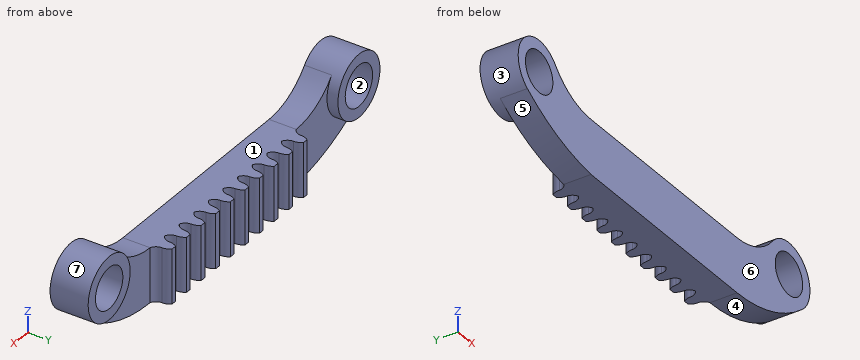
from build123d import *

# Parameters (mm, degrees)
SKETCH1_R                       = 3.75
BOSS_EXTRUDE1_DEPTH             = 5
BOSS_EXTRUDE2_REACH             = 43.932
SKETCH2_W                       = 1
SKETCH2_H                       = 1.5
BOSS_EXTRUDE2_DIRECTION_2_REACH = 43.932
LPATTERN1_COUNT                 = 10
LPATTERN1_PITCH                 = 4
SKETCH1_3_R                     = 5.75
SKETCH1_3_R_2                   = 3.75
BOSS_EXTRUDE3_DEPTH             = 7


with BuildPart() as part:
    # Sketch1 → Boss-Extrude1 (new body)
    with BuildSketch(Plane(origin=(0, 0, 0), x_dir=(1, 0, 0), z_dir=(0, 1, 0))):
        with BuildLine():
            ThreePointArc((-37.419913953, -1.242883661), (-38.427487159, -9.886669857), (-29.729020754, -9.627969703))
            ThreePointArc((-29.729020754, -9.627969703), (-25.386834609, -6.215943245), (-20, -5))
            Line((-20, -5), (20, -5))
            ThreePointArc((20, -5), (25.386834609, -6.215943245), (29.729020754, -9.627969703))
            ThreePointArc((29.729020754, -9.627969703), (38.202781159, -10.118262664), (37.932471123, -1.634635193))
            ThreePointArc((37.932471123, -1.634635193), (29.560228877, 3.288161479), (20, 5))
            Line((20, 5), (-20, 5))
            ThreePointArc((-20, 5), (-29.105909857, 2.983410588), (-37.419913953, -1.242883661))
        make_face()
        with Locations(Location((-34.19, -6, 0), (0, 0, 270))):
            Circle(SKETCH1_R, mode=Mode.SUBTRACT)
        with Locations(Location((34.19, -6, 0), (0, 0, 270))):
            Circle(SKETCH1_R, mode=Mode.SUBTRACT)
    extrude(amount=BOSS_EXTRUDE1_DEPTH)

    # Boss-Extrude2: up to this face of the body (flat: up to its plane)
    boss_extrude2_end = Plane(part.part.faces().sort_by_distance((0, 2.5, 5))[0])
    # Sketch2 → Boss-Extrude2 (add, up to the picked face)
    with BuildSketch(Plane.XY, mode=Mode.PRIVATE) as boss_extrude2_sk1:
        with BuildLine():
            ThreePointArc((-19, 6.5), (-19.272918272, 5.598612181), (-20, 5))
            Line((-20, 5), (-18, 5))
            Line((-18, 5), (-18, 6.5))
            Line((-18, 6.5), (-19, 6.5))
        make_face()
    boss_extrude2_tool1 = split(extrude(boss_extrude2_sk1.sketch, amount=BOSS_EXTRUDE2_REACH, mode=Mode.PRIVATE), bisect_by=boss_extrude2_end, keep=Keep.BOTH, mode=Mode.PRIVATE)
    # Sketch2 → Boss-Extrude2 (add, up to the picked face)
    with BuildSketch(Plane.XY, mode=Mode.PRIVATE) as boss_extrude2_sk2:
        with Locations((-17.5, 5.75)):
            Rectangle(SKETCH2_W, SKETCH2_H)
    boss_extrude2_tool2 = split(extrude(boss_extrude2_sk2.sketch, amount=BOSS_EXTRUDE2_REACH, mode=Mode.PRIVATE), bisect_by=boss_extrude2_end, keep=Keep.BOTH, mode=Mode.PRIVATE)
    # Sketch2 → Boss-Extrude2 (add, up to the picked face)
    with BuildSketch(Plane.XY, mode=Mode.PRIVATE) as boss_extrude2_sk3:
        with BuildLine():
            Line((-17, 6.5), (-17, 5))
            Line((-17, 5), (-16, 5))
            ThreePointArc((-16, 5), (-16.727081728, 5.598612181), (-17, 6.5))
        make_face()
    boss_extrude2_tool3 = split(extrude(boss_extrude2_sk3.sketch, amount=BOSS_EXTRUDE2_REACH, mode=Mode.PRIVATE), bisect_by=boss_extrude2_end, keep=Keep.BOTH, mode=Mode.PRIVATE)
    # Sketch2 → Boss-Extrude2 (add, up to the picked face)
    with BuildSketch(Plane.XY, mode=Mode.PRIVATE) as boss_extrude2_sk4:
        with BuildLine():
            Line((-18, 8), (-18, 6.5))
            Line((-18, 6.5), (-17, 6.5))
            ThreePointArc((-17, 6.5), (-17.128291755, 7.290569415), (-17.5, 8))
            Line((-17.5, 8), (-18, 8))
        make_face()
    boss_extrude2_tool4 = split(extrude(boss_extrude2_sk4.sketch, amount=BOSS_EXTRUDE2_REACH, mode=Mode.PRIVATE), bisect_by=boss_extrude2_end, keep=Keep.BOTH, mode=Mode.PRIVATE)
    # Sketch2 → Boss-Extrude2 (add, up to the picked face)
    with BuildSketch(Plane.XY, mode=Mode.PRIVATE) as boss_extrude2_sk5:
        with BuildLine():
            ThreePointArc((-18.5, 8), (-18.871708245, 7.290569415), (-19, 6.5))
            Line((-19, 6.5), (-18, 6.5))
            Line((-18, 6.5), (-18, 8))
            Line((-18, 8), (-18.5, 8))
        make_face()
    boss_extrude2_tool5 = split(extrude(boss_extrude2_sk5.sketch, amount=BOSS_EXTRUDE2_REACH, mode=Mode.PRIVATE), bisect_by=boss_extrude2_end, keep=Keep.BOTH, mode=Mode.PRIVATE)
    boss_extrude2_1 = boss_extrude2_tool1.solids().sort_by(Axis((-18.667854, 5.662777, 0), (0, 0, 1)))[0]
    add(boss_extrude2_1)
    boss_extrude2_2 = boss_extrude2_tool2.solids().sort_by(Axis((-17.5, 5.75, 0), (0, 0, 1)))[0]
    add(boss_extrude2_2)
    boss_extrude2_3 = boss_extrude2_tool3.solids().sort_by(Axis((-16.726983, 5.348311, 0), (0, 0, 1)))[0]
    add(boss_extrude2_3)
    boss_extrude2_4 = boss_extrude2_tool4.solids().sort_by(Axis((-17.56692, 7.177404, 0), (0, 0, 1)))[0]
    add(boss_extrude2_4)
    boss_extrude2_5 = boss_extrude2_tool5.solids().sort_by(Axis((-18.43308, 7.177404, 0), (0, 0, 1)))[0]
    add(boss_extrude2_5)
    boss_extrude2 = boss_extrude2_1 + boss_extrude2_2 + boss_extrude2_3 + boss_extrude2_4 + boss_extrude2_5  # Boss-Extrude2 as one shape, for the pattern or mirror that repeats it

    # Boss-Extrude2 direction 2: up to this face of the body (flat: up to its plane)
    boss_extrude2_direction_2_end = Plane(part.part.faces().sort_by_distance((0, 2.5, -5))[0])
    # Sketch2 → Boss-Extrude2 direction 2 (add, up to the picked face)
    with BuildSketch(Plane.XY, mode=Mode.PRIVATE) as boss_extrude2_direction_2_sk1:
        with BuildLine():
            ThreePointArc((-19, 6.5), (-19.272918272, 5.598612181), (-20, 5))
            Line((-20, 5), (-18, 5))
            Line((-18, 5), (-18, 6.5))
            Line((-18, 6.5), (-19, 6.5))
        make_face()
    boss_extrude2_direction_2_tool1 = split(extrude(boss_extrude2_direction_2_sk1.sketch, amount=-BOSS_EXTRUDE2_DIRECTION_2_REACH, mode=Mode.PRIVATE), bisect_by=boss_extrude2_direction_2_end, keep=Keep.BOTH, mode=Mode.PRIVATE)
    # Sketch2 → Boss-Extrude2 direction 2 (add, up to the picked face)
    with BuildSketch(Plane.XY, mode=Mode.PRIVATE) as boss_extrude2_direction_2_sk2:
        with Locations((-17.5, 5.75)):
            Rectangle(SKETCH2_W, SKETCH2_H)
    boss_extrude2_direction_2_tool2 = split(extrude(boss_extrude2_direction_2_sk2.sketch, amount=-BOSS_EXTRUDE2_DIRECTION_2_REACH, mode=Mode.PRIVATE), bisect_by=boss_extrude2_direction_2_end, keep=Keep.BOTH, mode=Mode.PRIVATE)
    # Sketch2 → Boss-Extrude2 direction 2 (add, up to the picked face)
    with BuildSketch(Plane.XY, mode=Mode.PRIVATE) as boss_extrude2_direction_2_sk3:
        with BuildLine():
            Line((-17, 6.5), (-17, 5))
            Line((-17, 5), (-16, 5))
            ThreePointArc((-16, 5), (-16.727081728, 5.598612181), (-17, 6.5))
        make_face()
    boss_extrude2_direction_2_tool3 = split(extrude(boss_extrude2_direction_2_sk3.sketch, amount=-BOSS_EXTRUDE2_DIRECTION_2_REACH, mode=Mode.PRIVATE), bisect_by=boss_extrude2_direction_2_end, keep=Keep.BOTH, mode=Mode.PRIVATE)
    # Sketch2 → Boss-Extrude2 direction 2 (add, up to the picked face)
    with BuildSketch(Plane.XY, mode=Mode.PRIVATE) as boss_extrude2_direction_2_sk4:
        with BuildLine():
            Line((-18, 8), (-18, 6.5))
            Line((-18, 6.5), (-17, 6.5))
            ThreePointArc((-17, 6.5), (-17.128291755, 7.290569415), (-17.5, 8))
            Line((-17.5, 8), (-18, 8))
        make_face()
    boss_extrude2_direction_2_tool4 = split(extrude(boss_extrude2_direction_2_sk4.sketch, amount=-BOSS_EXTRUDE2_DIRECTION_2_REACH, mode=Mode.PRIVATE), bisect_by=boss_extrude2_direction_2_end, keep=Keep.BOTH, mode=Mode.PRIVATE)
    # Sketch2 → Boss-Extrude2 direction 2 (add, up to the picked face)
    with BuildSketch(Plane.XY, mode=Mode.PRIVATE) as boss_extrude2_direction_2_sk5:
        with BuildLine():
            ThreePointArc((-18.5, 8), (-18.871708245, 7.290569415), (-19, 6.5))
            Line((-19, 6.5), (-18, 6.5))
            Line((-18, 6.5), (-18, 8))
            Line((-18, 8), (-18.5, 8))
        make_face()
    boss_extrude2_direction_2_tool5 = split(extrude(boss_extrude2_direction_2_sk5.sketch, amount=-BOSS_EXTRUDE2_DIRECTION_2_REACH, mode=Mode.PRIVATE), bisect_by=boss_extrude2_direction_2_end, keep=Keep.BOTH, mode=Mode.PRIVATE)
    boss_extrude2_direction_2_1 = boss_extrude2_direction_2_tool1.solids().sort_by(Axis((-18.667854, 5.662777, 0), (0, 0, -1)))[0]
    add(boss_extrude2_direction_2_1)
    boss_extrude2_direction_2_2 = boss_extrude2_direction_2_tool2.solids().sort_by(Axis((-17.5, 5.75, 0), (0, 0, -1)))[0]
    add(boss_extrude2_direction_2_2)
    boss_extrude2_direction_2_3 = boss_extrude2_direction_2_tool3.solids().sort_by(Axis((-16.726983, 5.348311, 0), (0, 0, -1)))[0]
    add(boss_extrude2_direction_2_3)
    boss_extrude2_direction_2_4 = boss_extrude2_direction_2_tool4.solids().sort_by(Axis((-17.56692, 7.177404, 0), (0, 0, -1)))[0]
    add(boss_extrude2_direction_2_4)
    boss_extrude2_direction_2_5 = boss_extrude2_direction_2_tool5.solids().sort_by(Axis((-18.43308, 7.177404, 0), (0, 0, -1)))[0]
    add(boss_extrude2_direction_2_5)
    boss_extrude2_direction_2 = boss_extrude2_direction_2_1 + boss_extrude2_direction_2_2 + boss_extrude2_direction_2_3 + boss_extrude2_direction_2_4 + boss_extrude2_direction_2_5  # Boss-Extrude2 direction 2 as one shape, for the pattern or mirror that repeats it

    # LPattern1: Boss-Extrude2, Boss-Extrude2 direction 2 ×10
    with Locations(*[(i * LPATTERN1_PITCH, 0, 0) for i in range(1, LPATTERN1_COUNT)]):
        add(boss_extrude2)
        add(boss_extrude2_direction_2)

    # Sketch1<3> → Boss-Extrude3 (add)
    # profile 1 of 2: a face of its own
    with BuildSketch(Plane(origin=(0, 0, 0), x_dir=(1, 0, 0), z_dir=(0, 1, 0))):
        with Locations(Location((-34.19, -6, 0), (0, 0, 124.175119346))):
            Circle(SKETCH1_3_R)
        with Locations(Location((-34.19, -6, 0), (0, 0, 270))):
            Circle(SKETCH1_3_R_2, mode=Mode.SUBTRACT)
    # profile 2 of 2: a face of its own
    with BuildSketch(Plane(origin=(0, 0, 0), x_dir=(1, 0, 0), z_dir=(0, 1, 0))):
        with Locations(Location((34.19, -6, 0), (0, 0, 49.393183525))):
            Circle(SKETCH1_3_R)
        with Locations(Location((34.19, -6, 0), (0, 0, 270))):
            Circle(SKETCH1_3_R_2, mode=Mode.SUBTRACT)
    extrude(amount=BOSS_EXTRUDE3_DEPTH)


solid = part.part
The listing builds one solid part. Answer for the finished solid, in the listing's coordinates (mm). Face numbers are marked on the shaded views. A direction names the side the tool comes from. Round coordinates to 2 decimals unless told otherwise and drop trailing zeros. Write each loop counter-clockwise with the first axis right and the second up, starting at its lowest first coordinate (ties: lowest second). Pieces come first, ordered by that corner, then holes. Notation, with made-up numbers: M 41.25,67 L 76.25,67 A28 cw 76.25,94 Z; hole C -19,30 d3. An arc over 180 degrees is marked long. Write each question's results on one line, items separated by ' | '. Start each with the question number.
Item 1: The mould has two halves that part along X. Classify the marked faces 4, 5, 6 and 7: +X half, -X half, draft (parallel to the pull), parting line (faces both ways), or undercut.
Item 2: Which of the six approach directions +Z, -Z, +X, -X, +Y, -Y give full straight-line access (tool end or side, diameter ignored) to the marked faces 1, 2 and 3?
Item 3: Find section B-B on z = 8. Write down the section's boundary in (x, y).
Item 4: Find section C-C on z = 3. Give the number of separate pieces and of enclosed holes in the cut face, and give its area (3 significant figures).
Item 5: Find section A-A on x = 34.19. Write down the section's boundary in (y, z).
Item 6: Given pin 1 Ø4 at (y, z) = (3.5, -1.5) entering from +X; pin 2 Ø7.5 at (x, z) = (-30.5, 3) entering from +Y; pin 3 Ø6 at (x, z) = (13, 6.5) entering from +Y; pin 4 Ø4 at (x, y) = (0, 4) entering from +Z, each flat-ended and moving along its own axis, determine where each tip first touches the part or whether it passes through.
Item 7: Find section D-D on x = -34.19. Write down the section's boundary in (y, z), and give its area (3 significant figures).
Item 8: Straight lines are drawn through the part: probe 1 along X at (y, z) = (3, 7.25); probe 2 along Y at (x, z) = (29.5, 7.5); probe 3 along Z at (x, y) = (-2.5, 5.5). For each, find the intervals that lie inside material, in ascending order.
Answer block:
1) face 4: +X half | face 5: -X half | face 6: draft | face 7: undercut
2) face 1: +Z, +Y, -Y | face 2: +Y, -Y | face 3: +Y
3) outline: M -39.58,0 L -37.36,0 L -37.36,7 L -39.58,7 Z; M -31.02,0 L -28.14,0 L -28.14,5 L -28.8,5 L -28.8,7 L -31.02,7 Z; M 28.14,0 L 31.02,0 L 31.02,7 L 28.8,7 L 28.8,5 L 28.14,5 Z; M 37.36,0 L 39.58,0 L 39.58,7 L 37.36,7 Z
4) separate pieces: 3 | enclosed holes: 0 | area: 431 mm²
5) outline: M 0,-1.06 L 5,-1.06 L 5,0.25 L 7,0.25 L 7,2.25 L 0,2.25 Z; M 0,9.75 L 7,9.75 L 7,11.75 L 0,11.75 Z
6) pin 1: stops at x = 36.52 | pin 2: stops at y = 7 | pin 3: stops at y = 8 | pin 4: stops at z = 5
7) outline: M 0,-0.72 L 5,-0.72 L 5,0.25 L 7,0.25 L 7,2.25 L 0,2.25 Z; M 0,9.75 L 7,9.75 L 7,11.75 L 0,11.75 Z | area: 32.8 mm²
8) probe 1: x = -39.8 to -37.73, -30.65 to -27.17, 27.17 to 30.65, 37.73 to 39.8 | probe 2: y = 0 to 7 | probe 3: z = -5 to 5
